Input: part model. Units: mm. Frame: model coordinates. Give positions to 0.01 mm unless a question says otherwise; leave off trailing zeros. Loops run counter-clockwise (first coordinate to the right, second up) from the corner with the lowest first, then second, coordinate; pieces in that order, holes last. Notation, with made-up numbers: (79.25, -31.75) - (129.25, -31.75) arc R25 cw to (129.25, 7.25) - close; hole circle Ø9 at (73, 73.25). An arc over 180 degrees is marked (long way). One line per item, written item: value.
from build123d import *

# Parameters (mm, degrees)
F0_W     = 3.5
F0_H     = 40
F0_W_2   = 5
F1_DEPTH = 3
F2_R     = 4.99999
F3_R     = 4.99999


# Not quite as in the source:
# - a fillet or chamfer is up to 0.001 mm smaller than in the source, because OpenCascade refuses the exact size


with BuildPart() as f1:
    # F0 (on Top) → F1 (new body)
    with BuildSketch(Plane.XY):
        Polygon((129.5, -200), (199, -200), (199, -157), (202, -157), (202, -117), (199, -117), (199, -77), (202, -77), (202, -37), (199, -37), (199, 6), (129.5, 6), (129.5, -37), (126, -37), (126, 6), (56.5, 6), (56.5, -37), (53, -37), (53, 6), (3, 6), (3, -37), (0, -37), (0, -77), (3, -77), (3, -117), (0, -117), (0, -157), (3, -157), (3, -200), (53, -200), (53, -157), (56.5, -157), (56.5, -200), (126, -200), (126, -157), (129.5, -157), align=None)
        Polygon((33, -134.75), (33, -137), (33, -139.25), (13, -139.25), (13, -134.75), align=None, mode=Mode.SUBTRACT)
        with Locations((54.75, -97)):
            Rectangle(F0_W, F0_H, mode=Mode.SUBTRACT)
        with Locations((127.75, -97)):
            Rectangle(F0_W, F0_H, mode=Mode.SUBTRACT)
        Polygon((134.5, -195), (134.5, -97), (134.5, 0), (194.5, 0), (194.5, -40), (184.5, -40), (184.5, -155), (194.5, -155), (194.5, -195), align=None, mode=Mode.SUBTRACT)
        with Locations((192, -97)):
            Rectangle(F0_W_2, F0_H, mode=Mode.SUBTRACT)
        Polygon((33, -54.75), (33, -57), (33, -59.25), (8.0116633326, -59.25), (8.0116633326, -54.75), align=None, mode=Mode.SUBTRACT)
    extrude(amount=F1_DEPTH)

    # F2 (radius 5 in the source; OpenCascade refuses exactly that, so slightly less here)
    f2_edges = [f1.edges().sort_by_distance(p)[0] for p in [
        (194.5, -40, 1.5),
        (184.5, -40, 1.5),
    ]]
    fillet(f2_edges, radius=F2_R)

    # F3 (radius 5 in the source; OpenCascade refuses exactly that, so slightly less here)
    f3_edges = [f1.edges().sort_by_distance(p)[0] for p in [
        (194.5, -155, 1.5),
        (184.5, -155, 1.5),
    ]]
    fillet(f3_edges, radius=F3_R)


solid = f1.part
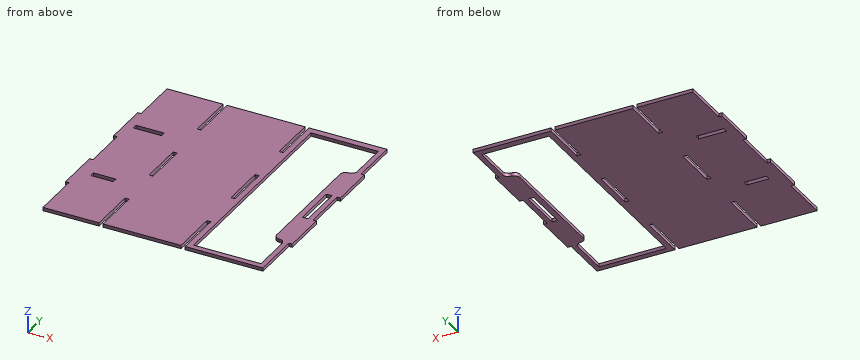
Item 1: Section C-C, the plane y = -179. Output: boundary loops of the cut face in (x, z), and give its area (3 significant figures).
Verdict:
outline: (3, 0) - (53, 0) - (53, 3) - (3, 3) - close; (56.5, 0) - (126, 0) - (126, 3) - (56.5, 3) - close; (129.5, 0) - (134.5, 0) - (134.5, 3) - (129.5, 3) - close; (194.5, 0) - (199, 0) - (199, 3) - (194.5, 3) - close
area: 387 mm^2
Item 2: Material intervals for L1, parallel to X at y = -162.5, z = 0.7; L2, parallel to X at y = -133.5, z = 0.35; L3, parallel to Y at x = 138, z = 0.65, sorted ascending.
Verdict:
L1: x = 3 to 53, 56.5 to 126, 129.5 to 134.5, 194.5 to 199
L2: x = 0 to 134.5, 184.5 to 202
L3: y = -200 to -195, 0 to 6
Item 3: Section B-B, the plane x = 22.5. Output: boundary loops of the cut face in (y, z), and give its area (3 significant figures).
Verdict:
outline: (-200, 0) - (-139.25, 0) - (-139.25, 3) - (-200, 3) - close; (-134.75, 0) - (-59.25, 0) - (-59.25, 3) - (-134.75, 3) - close; (-54.75, 0) - (6, 0) - (6, 3) - (-54.75, 3) - close
area: 591 mm^2
Item 4: Section D-D, the plane z = 2.25. Count the separate pieces of the cut face and the enclosed holes in it, and give its area (3 significant figures).
Verdict:
separate pieces: 1
enclosed holes: 6
area: 29,000 mm^2
Item 5: Pin query (flat end, axial travel): P1, Ø1.5, axis at x = 1.5, z = 1.5, coming from the -Y side; P2, Ø1.5, axis at x = 54, z = 1, coming from the +Y side; P3, Ø0.9, axis at y = -104.5, z = 1, coming from the +X side. Return the tip coordinate at first contact, or that it passes through.
Verdict:
P1: stops at y = -157
P2: stops at y = -37
P3: stops at x = 199
Item 6: Section A-A, the plane y = -124. Output: boundary loops of the cut face in (x, z).
Verdict:
outline: (0, 0) - (134.5, 0) - (134.5, 3) - (0, 3) - close; (184.5, 0) - (202, 0) - (202, 3) - (184.5, 3) - close
